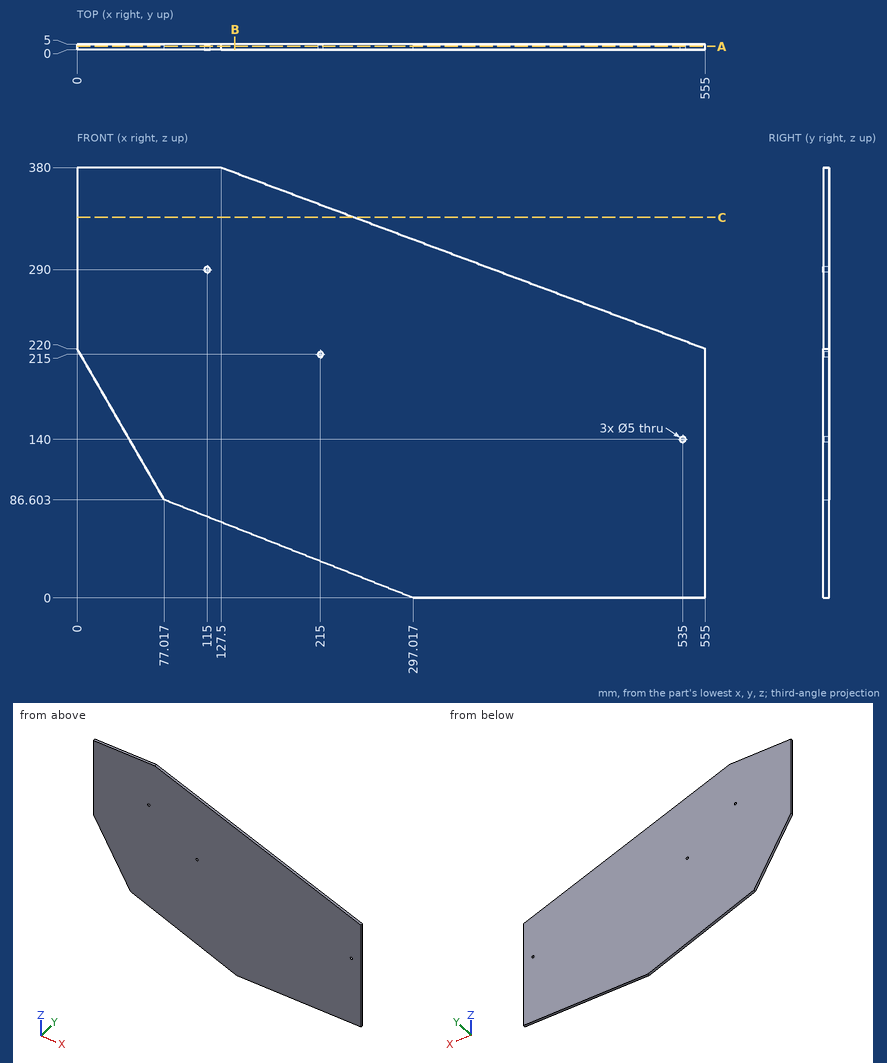
Verification items for this drawing (mm, ordinates from the low corner). Coordinates: 2 decimals unless noted, no trailing zeros. Loops run counter-clockwise (first coordinate to the right, second up) from the corner with the lowest first, then second, coordinate; pieces in that order, holes last. Notation, with made-up numbers: (77, -38) - (85, -38) arc R34 cw to (85, 1) - close; hole circle Ø10 at (2.25, 38.25). An arc over 180 degrees is marked (long way). Answer as a JSON object with one key per item and string values.
(1) Cross-section at A-A, the plane y = 3. Record the boundary of the cut face in (x, z).
Response:
{"outline": "(0, 220) - (77.02, 86.6) - (297.02, 0) - (555, 0) - (555, 220) - (127.5, 380) - (0, 380) - close; hole circle Ø5 at (115, 290); hole circle Ø5 at (215, 215); hole circle Ø5 at (535, 140)"}
(2) Scan lines: line 1 along X through (y, z) = (3.9, 140); line 2 along Z through (x, y) = (535, 4) (1 decimal); line 3 along Z through (x, y) = (115, 1). Record each from-to range of solid material in increasing order.
Response:
{"line 1": "x = 46.19 to 532.5, 537.5 to 555", "line 2": "z = 0 to 137.5, 142.5 to 227.5", "line 3": "z = 71.65 to 287.5, 292.5 to 380"}
(3) Cross-section at B-B, the plane x = 139.5. Record the boundary of the cut face in (y, z), then the cut area to 3 significant figures.
Response:
{"outline": "(0, 62.01) - (5, 62.01) - (5, 375.51) - (0, 375.51) - close", "area": "1,570 mm²"}
(4) Cross-section at C-C, the plane z = 336. Record the boundary of the cut face in (x, y).
Response:
{"outline": "(0, 0) - (245.06, 0) - (245.06, 5) - (0, 5) - close"}
(5) Go/stop test with flat-tipped pins: pin 1 Ø12 at (x, z) = (210.5, 271.5) entering from -Y; pin 2 Ø3 at (x, z) = (215, 215) entering from -Y. Record where each tip stops, or that it passes through.
Response:
{"pin 1": "stops at y = 0", "pin 2": "passes through"}
